Source: CAD feature listing. Evaluate the final solid. Frame: model axes, mm. A direction names the side the tool comes from. Coordinates: 2 decimals unless noted, no trailing zeros. Order: outer loops, then holes, each group sorted by start corner. A loop starts at its lowest first (then second) coordinate and runs counter-clockwise, first axis right, second up.
```python
from build123d import *

# Parameters (mm, degrees)
SKETCH1_W           = 60.5
SKETCH1_H           = 60.5
SKETCH1_R           = 15
SKETCH1_R_2         = 2.35
BOSS_EXTRUDE1_DEPTH = 6
SKETCH2_R           = 25.25
CUT_EXTRUDE1_DEPTH  = 3
SKETCH3_W           = 84.5
SKETCH3_H           = 55
BOSS_EXTRUDE2_DEPTH = 29.75
SKETCH4_W           = 55
SKETCH4_H           = 60.5
BOSS_EXTRUDE3_DEPTH = 12
SKETCH5_W           = 55
SKETCH5_H           = 60.5
BOSS_EXTRUDE4_DEPTH = 12
CHAMFER1_SIZE       = 3
SKETCH6_R           = 3.05
CUT_EXTRUDE2_DEPTH  = 30.75
SKETCH7_R           = 5.5
CUT_EXTRUDE3_DEPTH  = 7


with BuildPart() as part:
    # Sketch1 → Boss-Extrude1 (new body, symmetric)
    with BuildSketch(Plane.XY):
        Rectangle(SKETCH1_W, SKETCH1_H)
        Circle(SKETCH1_R, mode=Mode.SUBTRACT)
        with Locations((-25, 25)):
            Circle(SKETCH1_R_2, mode=Mode.SUBTRACT)
        with Locations((25, 25)):
            Circle(SKETCH1_R_2, mode=Mode.SUBTRACT)
        with Locations((25, -25)):
            Circle(SKETCH1_R_2, mode=Mode.SUBTRACT)
        with Locations((-25, -25)):
            Circle(SKETCH1_R_2, mode=Mode.SUBTRACT)
    extrude(amount=BOSS_EXTRUDE1_DEPTH, both=True)

    # Sketch2 → Cut-Extrude1 (cut)
    with BuildSketch(Plane.XY.offset(6)):
        Circle(SKETCH2_R)
    extrude(amount=-CUT_EXTRUDE1_DEPTH, mode=Mode.SUBTRACT)

    # Sketch3 → Boss-Extrude2 (add)
    with BuildSketch(Plane.XZ.offset(30.25)):
        with Locations((0, -3)):
            Rectangle(SKETCH3_W, SKETCH3_H)
    extrude(amount=BOSS_EXTRUDE2_DEPTH)

    # Sketch4 → Boss-Extrude3 (add)
    with BuildSketch(Plane(origin=(30.25, 0, 0), x_dir=(0, 0, -1), z_dir=(1, 0, 0))):
        with Locations((3, 0)):
            Rectangle(SKETCH4_W, SKETCH4_H)
    extrude(amount=BOSS_EXTRUDE3_DEPTH)

    # Sketch5 → Boss-Extrude4 (add)
    with BuildSketch(Plane.ZY.offset(30.25)):
        with Locations((-3, 0)):
            Rectangle(SKETCH5_W, SKETCH5_H)
    extrude(amount=BOSS_EXTRUDE4_DEPTH)

    # Chamfer1
    chamfer1_edges = [part.edges().sort_by_distance(p)[0] for p in [
        (36.25, 30.25, 24.5),
        (36.25, 30.25, -30.5),
        (-36.25, 30.25, -30.5),
        (-36.25, 30.25, 24.5),
    ]]
    chamfer(chamfer1_edges, length=CHAMFER1_SIZE)

    # Sketch6 → Cut-Extrude2 (cut, through all)
    with BuildSketch(Plane(origin=(0, -30.25, 0), x_dir=(1, 0, 0), z_dir=(0, 1, 0))):
        with Locations((0, -12.5)):
            Circle(SKETCH6_R)
        with Locations((-17.5, 18.5)):
            Circle(SKETCH6_R)
        with Locations((17.5, 18.5)):
            Circle(SKETCH6_R)
    extrude(amount=-CUT_EXTRUDE2_DEPTH, mode=Mode.SUBTRACT)

    # Sketch7 → Cut-Extrude3 (cut)
    with BuildSketch(Plane(origin=(0, -30.25, 0), x_dir=(1, 0, 0), z_dir=(0, 1, 0))):
        with Locations((-17.5, 18.5)):
            Circle(SKETCH7_R)
        with Locations((17.5, 18.5)):
            Circle(SKETCH7_R)
        with Locations((0, -12.5)):
            Circle(SKETCH7_R)
    extrude(amount=-CUT_EXTRUDE3_DEPTH, mode=Mode.SUBTRACT)


solid = part.part
```
1. Section query B-B, the plane y = 0. Output: boundary loops of the cut face in (x, z), plus the area to 3 significant figures.
2. Draft query along X for faces 1 (the cylindrical face through (23.135, -26.43, -0.084)), 2 (the flat face through (42.25, -14, -3)), 3 (the flat face through (-36.17, 28.77, 22.98)). Return one class per face: +X half, -X half, draft (parallel to the pull), parting line (faces both ways), or undercut.
3. Material intervals for line 1 along X through (y, z) = (-33.75, -18.5); line 2 along Y through (x, z) = (0, 0.75); line 3 along X through (y, z) = (4, 7.5), sorted ascending.
4. Section query A-A, the plane z = -18.5. Output: boundary loops of the cut face in (x, y), plus the area to 3 significant figures.
5. Access query for faces 4 (the flat face through (0, -30.25, -18)), 5 (the flat face through (20, -37.25, -16)), 6 (the flat face through (11, -11, 3)). Directions: +Z, -Z, +X, -X, +Y, -Y. A direction counts if a zero-diameter tool reaches every point of the face in a straight line with its end or side. Return the directions, or none.
6. Section query C-C, the plane z = 12.5. Output: boundary loops of the cut face in (x, y).
7. Contact query for flat-ended pins moving along their axis: P1, Ø12, axis at x = 24, y = 3.5, coming from the +Z side; P2, Ø1.5, axis at x = 12.5, y = -11, coming from the -Z side; P3, Ø9, axis at x = 18, z = -20, coming from the +Y side; P4, Ø6, axis at x = 28, y = -21, coming from the -Z side. Output: stop coordinate, or through.
8. Section query D-D, the plane y = -36. Output: boundary loops of the cut face in (x, z).
Answer key:
1. outline: (-42.25, -30.5) - (-30.25, -30.5) - (-30.25, -6) - (-15, -6) - (-15, 3) - (-25.25, 3) - (-25.25, 6) - (-30.25, 6) - (-30.25, 24.5) - (-42.25, 24.5) - close; (15, -6) - (30.25, -6) - (30.25, -30.5) - (42.25, -30.5) - (42.25, 24.5) - (30.25, 24.5) - (30.25, 6) - (25.25, 6) - (25.25, 3) - (15, 3) - close
1. area: 1,620 mm2
2. face 1: undercut
2. face 2: +X half
2. face 3: draft
3. line 1: x = -42.25 to -23, -12 to 12, 23 to 42.25
3. line 2: y = -60 to -15, 15 to 30.25
3. line 3: x = -42.25 to -30.25, 30.25 to 42.25
4. outline: (-42.25, -60) - (-20.55, -60) - (-20.55, -37.25) - (-23, -37.25) - (-23, -30.25) - (-30.25, -30.25) - (-30.25, 30.25) - (-42.25, 30.25) - close; (-14.45, -60) - (14.45, -60) - (14.45, -37.25) - (12, -37.25) - (12, -30.25) - (-12, -30.25) - (-12, -37.25) - (-14.45, -37.25) - close; (20.55, -60) - (42.25, -60) - (42.25, 30.25) - (30.25, 30.25) - (30.25, -30.25) - (23, -30.25) - (23, -37.25) - (20.55, -37.25) - close
4. area: 3,530 mm2
5. face 4: -Z, +Y
5. face 5: +Y
5. face 6: +Z
6. outline: (-42.25, -60) - (-3.05, -60) - (-3.05, -37.25) - (-5.5, -37.25) - (-5.5, -30.25) - (-30.25, -30.25) - (-30.25, 30.25) - (-42.25, 30.25) - close; (3.05, -60) - (42.25, -60) - (42.25, 30.25) - (30.25, 30.25) - (30.25, -30.25) - (5.5, -30.25) - (5.5, -37.25) - (3.05, -37.25) - close
7. P1: stops at z = 6
7. P2: stops at z = -6
7. P3: stops at y = -30.25
7. P4: stops at z = -30.5
8. outline: (-42.25, -30.5) - (42.25, -30.5) - (42.25, 24.5) - (-42.25, 24.5) - close; hole circle Ø11 at (-17.5, -18.5); hole circle Ø11 at (0, 12.5); hole circle Ø11 at (17.5, -18.5)
